from build123d import *

# Parameters (mm, degrees)
SKETCH_W             = 75
SKETCH_H             = 28.845
PAD_DEPTH            = 23.845
POCKET_DEPTH         = 24.076
POCKET001_DEPTH      = 24.076
SKETCH003_R          = 13.9225
POCKET002_DEPTH      = 19.076
SKETCH004_W          = 11.9225
SKETCH004_H          = 19.076
POCKET003_DEPTH      = 14.4235
POCKET003_DEPTH_BACK = -14.4235
SKETCH005_R          = 4
POCKET004_DEPTH      = 23.846
CHAMFER_SIZE         = 2
CHAMFER001_SIZE      = 1
SKETCH006_W          = 4.96125
SKETCH006_H          = 9.73025
POCKET005_DEPTH      = 29.845
SKETCH007_W          = 4.96125
SKETCH007_H          = 9.73025
POCKET006_DEPTH      = 29.845


with BuildPart() as part:
    # Sketch → Pad (new body)
    with BuildSketch(Plane.XY):
        Rectangle(SKETCH_W, SKETCH_H)
    extrude(amount=PAD_DEPTH)

    # Sketch001 → Pocket (cut)
    with BuildSketch(Plane.XZ.offset(-9.6535)):
        Polygon((0, 4.769), (-35.5, 4.769), (-35.5, 8.538), (0, 19.076), align=None)
    extrude(amount=POCKET_DEPTH, mode=Mode.SUBTRACT)

    # Sketch002 → Pocket001 (cut)
    with BuildSketch(Plane.XZ.offset(9.6535)):
        Polygon((0, 4.769), (0, 19.076), (35.5, 8.538), (35.5, 4.769), align=None)
    extrude(amount=-POCKET001_DEPTH, mode=Mode.SUBTRACT)

    # Sketch003 → Pocket002 (cut)
    with BuildSketch(Plane.XY.offset(23.845)):
        Circle(SKETCH003_R)
    extrude(amount=-POCKET002_DEPTH, mode=Mode.SUBTRACT)

    # Sketch004 → Pocket003 (cut, two sides)
    with BuildSketch(Plane.XZ) as pocket003_sk:
        with Locations((0, 14.307)):
            Rectangle(SKETCH004_W, SKETCH004_H)
    extrude(amount=-POCKET003_DEPTH, mode=Mode.SUBTRACT)
    extrude(pocket003_sk.sketch, amount=-POCKET003_DEPTH_BACK, mode=Mode.SUBTRACT)

    # Sketch005 → Pocket004 (cut, through all)
    with BuildSketch(Plane.XY.offset(23.845)):
        with Locations((-21.5, 0)):
            Circle(SKETCH005_R)
        with Locations((21.5, 0)):
            Circle(SKETCH005_R)
    extrude(amount=-POCKET004_DEPTH, mode=Mode.SUBTRACT)

    # Chamfer
    chamfer_edges = [part.edges().sort_by_distance(p)[0] for p in [
        (-25.5, 0, 4.769),
        (17.5, 0, 4.769),
    ]]
    chamfer(chamfer_edges, length=CHAMFER_SIZE)

    # Chamfer001
    chamfer001_edges = [part.edges().sort_by_distance(p)[0] for p in [
        (21.730625, 14.4225, 23.845),
        (-21.730625, 14.4225, 23.845),
        (21.730625, -14.4225, 23.845),
        (-21.730625, -14.4225, 23.845),
        (-37.5, 0, 23.845),
        (37.5, 0, 23.845),
        (20.730625, 14.4225, 4.769),
        (-20.730625, -14.4225, 4.769),
        (-37.5, -14.4225, 11.9225),
        (37.5, 14.4225, 11.9225),
        (37.5, -14.4225, 11.9225),
        (-37.5, 14.4225, 11.9225),
    ]]
    chamfer(chamfer001_edges, length=CHAMFER001_SIZE)

    # Sketch006 → Pocket005 (cut)
    with BuildSketch(Plane.XZ):
        with Locations((-7.441875, 19.979875)):
            Rectangle(SKETCH006_W, SKETCH006_H)
    extrude(amount=POCKET005_DEPTH, mode=Mode.SUBTRACT)

    # Sketch007 → Pocket006 (cut)
    with BuildSketch(Plane.XZ):
        with Locations((7.441875, 19.979875)):
            Rectangle(SKETCH007_W, SKETCH007_H)
    extrude(amount=-POCKET006_DEPTH, mode=Mode.SUBTRACT)


solid = part.part
Input: part model. Units: mm. Frame: model coordinates. A direction names the side the tool comes from. Round coordinates to 2 decimals unless told otherwise and drop trailing zeros. Order: outer loops, then holes, each group sorted by start corner. A loop starts at its lowest first (then second) coordinate and runs counter-clockwise, first axis right, second up. Notation, with made-up numbers: (-7, 84) - (6, 84) arc R14 ccw to (6, 97) - close; hole circle Ø9 at (-28.75, 66.5). An arc over 180 degrees is marked (long way). Use a Markdown table: item, result.
1. Material intervals for probe 1 along X at (y, z) = (0, 22); probe 2 along X at (y, z) = (1.5, 4); probe 3 along Y at (x, z) = (-21.5, 1.2), sorted ascending.
Evaluation:
| item | result |
|---|---|
| probe 1 | -37.5 to -25.5, -17.5 to -13.92, 13.92 to 17.5, 25.5 to 37.5 |
| probe 2 | -37.5 to -26.51, -16.49 to 16.49, 26.51 to 37.5 |
| probe 3 | -14.42 to -4, 4 to 14.42 |
2. Access query for faces 1 (the face through (-22, 4.1, 2.9)), 2 (the face through (12.82, -5.43, 18.68)), 3 (the face through (20, -9.654, 9)), 4 (the face through (9.922, 12, 20)), 5 (the face through (-9.922, -12, 20)). Directions: +Z, -Z, +X, -X, +Y, -Y. A direction counts if a zero-diameter tool reaches every point of the face in a straight line with its end or side. Return the directions, or none.
Evaluation:
| item | result |
|---|---|
| face 1 | none |
| face 2 | +Z |
| face 3 | +Y |
| face 4 | +Z, +Y |
| face 5 | +Z, -Y |
3. Section A-A on z = 19.25. Return the cut outline in (x, y) (1 decimal).
Evaluation:
| item | result |
|---|---|
| outline | (-37.5, -13.4) - (-36.5, -14.4) - (-9.9, -14.4) - (-9.9, -9.8) arc R13.9 cw to (-6, 12.6) - (-6, 14.4) - (-36.5, 14.4) - (-37.5, 13.4) - close; (6, -14.4) - (36.5, -14.4) - (37.5, -13.4) - (37.5, 13.4) - (36.5, 14.4) - (9.9, 14.4) - (9.9, 9.8) arc R13.9 cw to (6, -12.6) - close; hole circle Ø8 at (-21.5, 0); hole circle Ø8 at (21.5, 0) |
4. Mould query, pull axis Z, two halves, no side actions, for faces 6 (the face through (-20, 9.654, 9)), 7 (the face through (-1, 0, 0)), 8 (the face through (-25, 3, 23.845)). Classes: +Z half, -Z half, draft (parallel to the pull), parting line (faces both ways), or undercut.
Evaluation:
| item | result |
|---|---|
| face 6 | undercut |
| face 7 | -Z half |
| face 8 | +Z half |
5. First-contact query: pin 1 (10.5 mm diameter, centred on x = -21.5, y = 0, fed in from +Z) (3 decimals); pin 2 (8 mm diameter, centred on x = 9.5, y = 2, fed in from +Z); pin 3 (6.5 mm diameter, centred on x = 21.5, y = 0, fed in from -Z). Flat tips, straight axial feed; report the tip coordinate or a pass-through.
Evaluation:
| item | result |
|---|---|
| pin 1 | z = 23.845 |
| pin 2 | z = 4.77 |
| pin 3 | through |
6. Section B-B on z = 2. Return the cut outline in (x, y), then the cut area to 3 significant figures.
Evaluation:
| item | result |
|---|---|
| outline | (-37.5, -13.42) - (-36.5, -14.42) - (36.5, -14.42) - (37.5, -13.42) - (37.5, 13.42) - (36.5, 14.42) - (-36.5, 14.42) - (-37.5, 13.42) - close; hole circle Ø8 at (-21.5, 0); hole circle Ø8 at (21.5, 0) |
| area | 2,060 mm^2 |
7. Section D-D on x = 21.5. Return the cut outline in (y, z) (1 decimal).
Evaluation:
| item | result |
|---|---|
| outline | (-14.4, 0) - (-4, 0) - (-4, 2.8) - (-6, 4.8) - (-9.7, 4.8) - (-9.7, 12.7) - (-4, 12.7) - (-4, 23.8) - (-13.4, 23.8) - (-14.4, 22.8) - close; (4, 0) - (14.4, 0) - (14.4, 3.8) - (13.4, 4.8) - (6, 4.8) - (4, 2.8) - close; (4, 12.7) - (14.4, 12.7) - (14.4, 22.8) - (13.4, 23.8) - (4, 23.8) - close |
8. Section C-C on y = 0. State how many separate pieces and enclosed holes the cut face has, then the cut area to 3 significant figures.
Evaluation:
| item | result |
|---|---|
| separate pieces | 5 |
| enclosed holes | 0 |
| area | 693 mm^2 |
